Could you check a few things on this drawing? It's one solid part, dimensions in mm from its lowest x, y, z. A direction names the side the tool comes from. Give positions to 0.01 mm unless a question says otherwise; leave off trailing zeros. Write each loop counter-clockwise with the first axis right and the second up, starting at its lowest first coordinate (ties: lowest second). Pieces come first, ordered by that corner, then holes. Notation, with made-up numbers: M 31.25,89 L 40.25,89 A23 cw 40.25,97 Z; hole C -2,50 d9. An arc over 180 degrees is marked long. Answer as CSV lines item,"result". Start each with the question number.
Q1. For pin 1 (2.5 mm diameter, centred on x = 3, z = 3, fed in from +Y), with a flat end and sliding along its axis, tell me the tip position at first contact or that it passes through.
Q2. Suppose I cut it at C-C (z = 3). Write out the boundary of the cut face in (x, y), then the cut area to 4 significant figures.
Q3. Suppose I cut it at B-B (y = 7.75). Write out the boundary of the cut face in (x, z), then the cut area to 3 significant figures.
Q4. Suppose I cut it at D-D (z = 1.1). Write out the boundary of the cut face in (x, y), then the cut area to 3 significant figures.
Q5. If I drill on line 1 along Y through (x, z) = (3.95, 1.55); line 2 along X through (y, z) = (7, 3); line 3 along Y through (x, z) = (4.25, 4.35), over which ranges is the centre line in solid material (lowest first)?
Q6. On a 3-axis mill with a long thin cutter (end or side, diameter ignored), from which of +Z, -Z, +X, -X, +Y, -Y can I reach the whole of each face in a straight line? I mean the marked faces 1, 2, 3 and 4. Say none if no direction works.
Q7. Suppose I cut it at A-A (x = 3). Write out the boundary of the cut face in (y, z), then the cut area to 4 significant figures.
Q8. Thinking about a two-plate mould opening in Y: for the marked faces 5, 6 and 7, which applies, +Y half, -Y half, draft (parallel to the pull), parting line (faces both ways), or undercut?
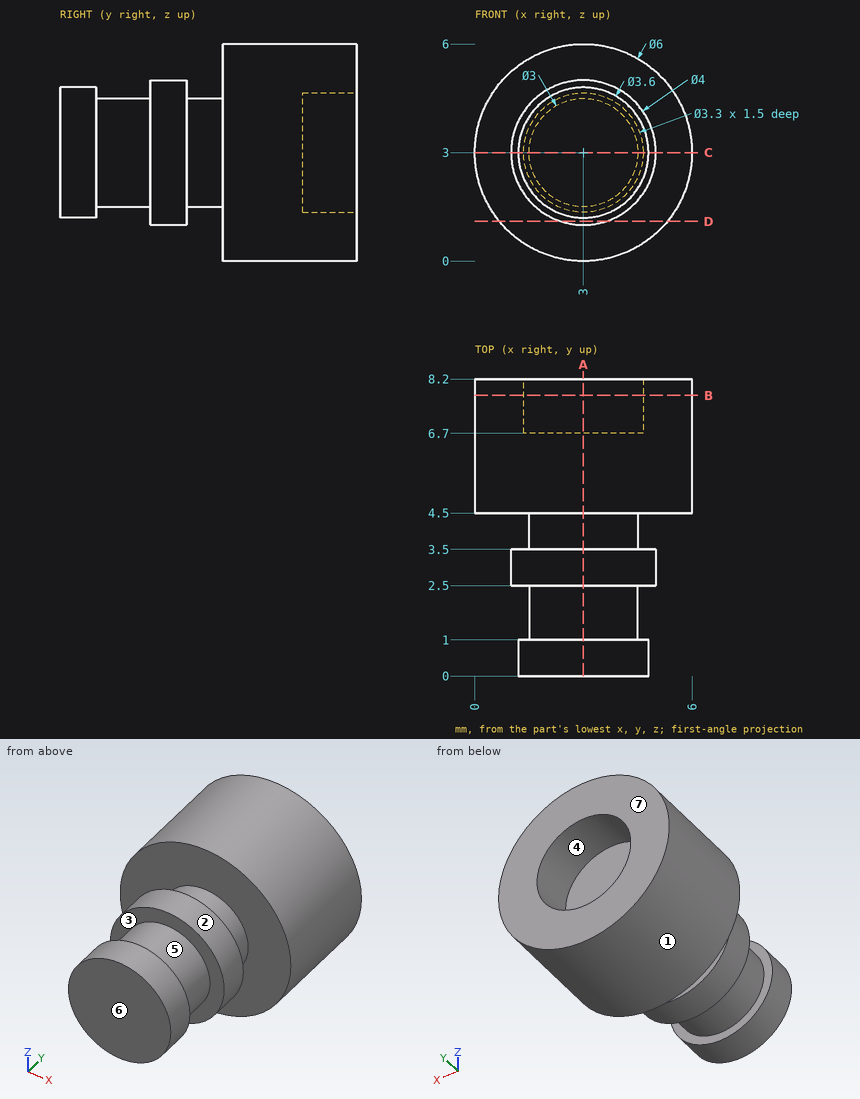
Resolved:
1,pin 1,"y = 6.7"
2,outline,"M 0,4.5 L 1.5,4.5 L 1.5,3.5 L 1,3.5 L 1,2.5 L 1.5,2.5 L 1.5,1 L 1.2,1 L 1.2,0 L 4.8,0 L 4.8,1 L 4.5,1 L 4.5,2.5 L 5,2.5 L 5,3.5 L 4.5,3.5 L 4.5,4.5 L 6,4.5 L 6,8.2 L 4.65,8.2 L 4.65,6.7 L 1.35,6.7 L 1.35,8.2 L 0,8.2 Z"
2,area,"32.35 mm^2"
3,outline,"C 3,3 d6; hole C 3,3 d3.3"
3,area,"19.7 mm^2"
4,outline,"M 0.68,4.5 L 5.32,4.5 L 5.32,8.2 L 0.68,8.2 Z; M 2.38,2.5 L 3.62,2.5 L 3.62,3.5 L 2.38,3.5 Z"
4,area,"18.4 mm^2"
5,line 1,"0 to 1, 2.5 to 3.5, 4.5 to 8.2"
5,line 2,"0 to 1.35, 4.65 to 6"
5,line 3,"2.5 to 3.5, 4.5 to 8.2"
6,face 1,"+Y, -Y"
6,face 2,"-Y"
6,face 3,"none"
6,face 4,"+Y"
7,outline,"M 0,1.2 L 1,1.2 L 1,1.5 L 2.5,1.5 L 2.5,1 L 3.5,1 L 3.5,1.5 L 4.5,1.5 L 4.5,0 L 8.2,0 L 8.2,1.35 L 6.7,1.35 L 6.7,4.65 L 8.2,4.65 L 8.2,6 L 4.5,6 L 4.5,4.5 L 3.5,4.5 L 3.5,5 L 2.5,5 L 2.5,4.5 L 1,4.5 L 1,4.8 L 0,4.8 Z"
7,area,"32.35 mm^2"
8,face 5,"undercut"
8,face 6,"-Y half"
8,face 7,"+Y half"
